from build123d import *

# Parameters (mm, degrees)
F1_DEPTH = 19.05
F2_W     = 152.4
F2_H     = 31.75
F2_W_2   = 31.75
F2_H_2   = 152.4
F3_DEPTH = 6.35
F4_D     = 5


with BuildPart() as f1:
    # F0 (on Top) → F1 (new body)
    with BuildSketch(Plane.XY):
        Polygon((-9.525, -155.575), (-224.8118673418, -155.575), (-224.8118673418, -174.625), (224.8118673418, -174.625), (224.8118673418, -155.575), (9.525, -155.575), (9.525, 280.162), (-9.525, 280.162), align=None)
    extrude(amount=F1_DEPTH)

    # F2 (on face) → F3 (join)
    with BuildSketch(Plane.XY.offset(19.05)):
        with Locations((0, -158.75)):
            Rectangle(F2_W, F2_H)
        Rectangle(F2_W_2, F2_H_2)
    extrude(amount=F3_DEPTH)

    # F4 (through all)
    with Locations(Plane(origin=(0, 0, 0), x_dir=(1, 0, 0), z_dir=(0, 0, -1))):
        with Locations((186.7118673418, 165.1), (0, -249.2375), (-186.7118673418, 165.1), (-217.4817061272, 165.1), (217.4817061272, 165.1), (0, -273.05)):
            Hole(F4_D / 2)


solid = f1.part
CAD build for the part. Positions are in the model's coordinates, mm. A direction names the side the tool comes from. Coordinates: 2 decimals unless noted, no trailing zeros. Write each loop counter-clockwise with the first axis right and the second up, starting at its lowest first coordinate (ties: lowest second). Pieces come first, ordered by that corner, then holes. Notation, with made-up numbers: (70.5, 5) - (98.5, 5) arc R31 ccw to (98.5, 39) - close; hole circle Ø6 at (76, 59.25). An arc over 180 degrees is marked (long way). Use a Markdown table: item, result. Add a question column.
Item 1: Band-saw the part on A-A, the plane y = 33. Give the cut face in (x, z) (3 decimals).
Item 2: Band-saw the part on D-D, the plane y = 177. Give the cut face in (x, z) (3 decimals).
Item 3: Flat gauge pins, fed straight in: pin 1 (5.5 mm diameter, centred on y = -33.5, z = 12.5, fed in from +X) (3 decimals); pin 2 (7 mm diameter, centred on y = 3.5, z = 22.5, fed in from +X) (3 decimals); pin 3 (21 mm diameter, centred on x = 4.5, y = -111.5, fed in from +Z); pin 4 (7 mm diameter, centred on y = -166, z = 22, fed in from +X). Where does each tip first touch, or does it go through?
Item 4: 3-axis set-ups, long thin cutter, end or side, ignore diameter. For faces 1 (the face through (-152, -165, 19.05)), 2 (the face through (9.525, 59, 9)), 3 (the face through (149, -165, 19.05)), 4 (the face through (-116, -155.575, 9)), 5 (the face through (0, 180, 19.05)): which of +Z, -Z, +X, -X, +Y, -Y reach the whole face in a straight line?
Item 5: Drill centre lines: L1, parallel to X at y = -165.1, z = 4; L2, parallel to X at y = 273.05, z = 4.75 (3 decimals); L3, parallel to X at y = 78, z = 13.25 (3 decimals). Where is each one in solid material? Low to high. Write a range as from..to.
Item 6: Band-saw the part on C-C, the plane x = -57.5. Give the cut face in (y, z) (3 decimals), and give its area (3 significant figures).
Item 7: Band-saw the part on B-B, the plane z = 4. Give the number of separate pieces and of enclosed holes in the cut face, and give its area (3 significant figures).
Numbers:
| question | item | result |
|---|---|---|
| 1 | outline | (-15.875, 19.05) - (-9.525, 19.05) - (-9.525, 0) - (9.525, 0) - (9.525, 19.05) - (15.875, 19.05) - (15.875, 25.4) - (-15.875, 25.4) - close |
| 2 | outline | (-9.525, 0) - (9.525, 0) - (9.525, 19.05) - (-9.525, 19.05) - close |
| 3 | pin 1 | x = 9.525 |
| 3 | pin 2 | x = 15.875 |
| 3 | pin 3 | z = 19.05 |
| 3 | pin 4 | x = 224.81 |
| 4 | face 1 | +Z, -X, +Y, -Y |
| 4 | face 2 | -Z, +X, +Y |
| 4 | face 3 | +Z, +X, +Y, -Y |
| 4 | face 4 | -Z, -X, +Y |
| 4 | face 5 | +Z, +X, -X, +Y |
| 5 | L1 | -224.81..-219.98, -214.98..-189.21, -184.21..184.21, 189.21..214.98, 219.98..224.81 |
| 5 | L2 | -9.525..-2.5, 2.5..9.525 |
| 5 | L3 | -9.525..9.525 |
| 6 | outline | (-174.625, 0) - (-155.575, 0) - (-155.575, 19.05) - (-142.875, 19.05) - (-142.875, 25.4) - (-174.625, 25.4) - close |
| 6 | area | 565 mm2 |
| 7 | separate pieces | 1 |
| 7 | enclosed holes | 6 |
| 7 | area | 16,700 mm2 |
